```python
from build123d import *

# Parameters (mm, degrees)
F0_W     = 178
F0_H     = 80
F1_DEPTH = 70
F3_DEPTH = 69
F4_R     = 5
F5_R     = 0.49999


# Not quite as in the source:
# - a fillet or chamfer is up to 0.001 mm smaller than in the source, because OpenCascade refuses the exact size


with BuildPart() as f1:
    # F0 (on Top) → F1 (new body)
    with BuildSketch(Plane.XY):
        Rectangle(F0_W, F0_H)
    extrude(amount=F1_DEPTH)

    # F2 (on face) → F3 (cut)
    with BuildSketch(Plane.XY.offset(70)):
        Polygon((-88, -24.0239519626), (-88, -39), (-83.0030292273, -39), (89, -39), (89, 39), (-88, 39), align=None)
    extrude(amount=-F3_DEPTH, mode=Mode.SUBTRACT)

    # F4
    f4_edges = [f1.edges().sort_by_distance(p)[0] for p in [
        (-88, 39, 35.5),
        (0.5, 39, 1),
        (-88, 0, 1),
        (-88, -39, 35.5),
        (0.5, -39, 1),
        (0, 40, 0),
        (-89, 40, 35),
        (-89, -40, 35),
        (0, -40, 0),
    ]]
    fillet(f4_edges, radius=F4_R)

    # F5 (radius 0.5 in the source; OpenCascade refuses exactly that, so slightly less here)
    f5_edges = [f1.edges().sort_by_distance(p)[0] for p in [
        (-89, 0, 70),
        (-87.535534, 38.535534, 70),
        (-87.535534, -38.535534, 70),
        (2.5, 40, 70),
        (2.5, -40, 70),
        (89, 39.5, 70),
        (89, -39.5, 70),
        (3, 39, 70),
        (3, -39, 70),
        (-86.535534, 37.535534, 70),
        (-86.535534, -37.535534, 70),
        (-88, 0, 70),
    ]]
    fillet(f5_edges, radius=F5_R)


solid = f1.part
```
Input: part model. Units: mm. Frame: model coordinates. A direction names the side the tool comes from. Round coordinates to 2 decimals unless told otherwise and drop trailing zeros. Write each loop counter-clockwise with the first axis right and the second up, starting at its lowest first coordinate (ties: lowest second). Pieces come first, ordered by that corner, then holes. Notation, with made-up numbers: (-6.75, 1.5) -> (7.25, 1.5) arc R23 cw to (7.25, 21.5) -> close; hole circle Ø9 at (2.25, 72). An arc over 180 degrees is marked (long way). Answer as CSV lines item,"result".
1. Contact query for flat-ended pins moving along their axis: P1, Ø19, axis at y = -11, z = 34, coming from the +X side; P2, Ø6, axis at x = 34.5, y = -5, coming from the +Z side. Output: stop coordinate, or through.
Geometry says:
P1,"stops at x = -88"
P2,"stops at z = 1"
2. Mould query, pull axis Y, two halves, no side actions, for faces 3 (the flat face through (2, -39, 38)), 4 (the cylindrical face through (1, 39, 2)), 5 (the cylindrical face through (-88, -38, 35)), 6 (the cylindrical face through (2, 38, 3)). Classes: +Y half, -Y half, draft (parallel to the pull), parting line (faces both ways), or undercut.
Geometry says:
face 3,"undercut"
face 4,"+Y half"
face 5,"-Y half"
face 6,"undercut"
3. Reachability of faces 1 (the cylindrical face through (4, -38, 3)), 2 (the flat face through (1, 40, 37)) from +Z, -Z, +X, -X, +Y, -Y: full face, straight path, thin tool, end or side. Return the list, or none.
Geometry says:
face 1,"+Z, +X"
face 2,"+Z, -Z, +X, -X, +Y"
4. Section B-B (z = 15.5). Return the cut outline in (x, y), plus the area to 3 significant figures.
Geometry says:
outline,"(-89, -35) arc R5 ccw to (-84, -40) -> (89, -40) -> (89, -39) -> (-83, -39) arc R5 cw to (-88, -34) -> (-88, 34) arc R5 cw to (-83, 39) -> (89, 39) -> (89, 40) -> (-84, 40) arc R5 ccw to (-89, 35) -> close"
area,"434 mm^2"
5. Ray query, L1, parallel to Y at x = -55.5, z = 53.5; L2, parallel to Z at x = -65, y = 18; L3, parallel to X at y = 16, z = 13. Return the intervals inside material, ascending. Write a range as [from, to].
Geometry says:
L1,"y = [-40, -39], [39, 40]"
L2,"z = [0, 1]"
L3,"x = [-89, -88]"
